from build123d import *

# Parameters (mm, degrees)
SKETCH1_W           = 127
SKETCH1_H           = 76.2
SKETCH1_R           = 8.33021032
SKETCH1_R_2         = 12.7
SKETCH1_W_2         = 8.659801889
SKETCH1_H_2         = 17.712025184
BOSS_EXTRUDE1_DEPTH = 25.4


with BuildPart() as part:
    # Sketch1 → Boss-Extrude1 (new body)
    with BuildSketch(Plane(origin=(0, 0, 0), x_dir=(1, 0, 0), z_dir=(0, 1, 0))):
        with Locations((63.5, 38.1)):
            Rectangle(SKETCH1_W, SKETCH1_H)
        with Locations(Location((68.491601229, 24.568808003, 0), (0, 0, 270))):
            Circle(SKETCH1_R, mode=Mode.SUBTRACT)
        with Locations(Location((101.6, 50.8, 0), (0, 0, 270))):
            Circle(SKETCH1_R_2, mode=Mode.SUBTRACT)
        with Locations((41.585480672, 24.535685835)):
            Rectangle(SKETCH1_W_2, SKETCH1_H_2, mode=Mode.SUBTRACT)
    extrude(amount=BOSS_EXTRUDE1_DEPTH)

    # Mirror1: part across plane


with BuildPart() as part_1:
    add(part.part)
    add(part.part.mirror(Plane(origin=(0, 25.4, 0), x_dir=(0, 0, 1), z_dir=(1, 0, 0))))

    # Mirror2: part across plane


with BuildPart() as part_2:
    add(part_1.part)
    add(part_1.part.mirror(Plane(origin=(0, 25.4, 0), x_dir=(1, 0, 0), z_dir=(0, 0, -1))))

    # Mirror3: part across face


with BuildPart() as part_3:
    add(part_2.part)
    add(part_2.part.mirror(Plane(origin=(0, 12.7, 76.2), x_dir=(1, 0, 0), z_dir=(0, 0, 1))))


solid = part_3.part
CAD build for the part. Positions are in the model's coordinates, mm. A direction names the side the tool comes from. Round coordinates to 2 decimals unless told otherwise and drop trailing zeros. Write each loop counter-clockwise with the first axis right and the second up, starting at its lowest first coordinate (ties: lowest second). Pieces come first, ordered by that corner, then holes.
(1) Slice it at A-A, the plane x = 101.6. Write the cut outline in (y, z), and give its area (3 significant figures).
(2) 3-axis set-ups, long thin cutter, end or side, ignore diameter. For faces 1 (the face through (-127, 13, 78)), 2 (the face through (-42, 13, 168.08)): which of +Z, -Z, +X, -X, +Y, -Y reach the whole face in a straight line?
(3) Probe line 1 along X through (y, z) = (16.75, 203.2); line 2 along X through (y, z) = (15, 49.5); line 3 along Z through (x, y) = (-39.5, 17). List the from-to ranges inside material, lowest first.
(4) Drop flat-ended pins along their axis: P1, Ø19, axis at x = -68.49, z = 127.83, coming from the -Y side; P2, Ø15, axis at x = 101.6, z = 50.8, coming from the -Y side. Give the stop position or say it passes through.
(5) Mould opens along Z. For faces 3 (the face through (2, 13, -76.2)), 4 (the face through (37.256, 13, 128)), 5 (the face through (2, 25.4, 74)) say: pulls with the +Z half, pulls with the -Z half, needs draft (parallel to the pull), parting line crosses it, or undercut.
(6) Slice it at C-C, the plane z = 26.5. Write the cut outline in (x, y).
(7) Slice it at D-D, the plane y = 15.75. Count the separate pieces of the cut face and the enclosed holes in it, and give its area (3 significant figures).
(8) Slice it at B-B, the plane z = -50.8. Write the cut outline in (x, y), and give its area (3 significant figures).
From the geometry:
1. outline: (0, -76.2) - (25.4, -76.2) - (25.4, -63.5) - (0, -63.5) - close; (0, -38.1) - (25.4, -38.1) - (25.4, 38.1) - (0, 38.1) - close; (0, 63.5) - (25.4, 63.5) - (25.4, 88.9) - (0, 88.9) - close; (0, 114.3) - (25.4, 114.3) - (25.4, 190.5) - (0, 190.5) - close; (0, 215.9) - (25.4, 215.9) - (25.4, 228.6) - (0, 228.6) - close
1. area: 5,160 mm2
2. face 1: +Z, -Z, -X, +Y, -Y
2. face 2: +Y, -Y
3. line 1: x = -127 to -114.3, -88.9 to 88.9, 114.3 to 127
3. line 2: x = -127 to -114.23, -88.97 to 88.97, 114.23 to 127
3. line 3: z = -76.2 to -33.39, -15.68 to 15.68, 33.39 to 119.01, 136.72 to 168.08, 185.79 to 228.6
4. P1: stops at y = 0
4. P2: passes through
5. face 3: pulls with the -Z half
5. face 4: undercut
5. face 5: needs draft
6. outline: (-127, 0) - (-76.59, 0) - (-76.59, 25.4) - (-127, 25.4) - close; (-60.39, 0) - (-45.92, 0) - (-45.92, 25.4) - (-60.39, 25.4) - close; (-37.26, 0) - (37.26, 0) - (37.26, 25.4) - (-37.26, 25.4) - close; (45.92, 0) - (60.39, 0) - (60.39, 25.4) - (45.92, 25.4) - close; (76.59, 0) - (127, 0) - (127, 25.4) - (76.59, 25.4) - close
7. separate pieces: 1
7. enclosed holes: 24
7. area: 70,400 mm2
8. outline: (-127, 0) - (-114.3, 0) - (-114.3, 25.4) - (-127, 25.4) - close; (-88.9, 0) - (88.9, 0) - (88.9, 25.4) - (-88.9, 25.4) - close; (114.3, 0) - (127, 0) - (127, 25.4) - (114.3, 25.4) - close
8. area: 5,160 mm2
